from build123d import *

# Parameters (mm, degrees)
F0_W     = 165.1
F0_H     = 304.8
F0_W_2   = 139.7
F0_H_2   = 152.4
F0_W_3   = 127
F0_H_3   = 121.92
F0_W_4   = 88.9
F0_H_4   = 114.3
F1_DEPTH = 50.8
F2_DEPTH = 5
F3_DEPTH = 38.1
F4_R     = 10
F5_R     = 3.81
F6_DEPTH = 129.54


# Not quite as in the source:
# - a feature names something its author has since deleted; it is built from what else it names


with BuildPart() as f1:
    # F0 (on Front) → F1 (new body)
    with BuildSketch(Plane.XZ):
        with Locations((0, -38.1)):
            Rectangle(F0_W, F0_H)
        Rectangle(F0_W_2, F0_H_2, mode=Mode.SUBTRACT)
        Rectangle(F0_W_2, F0_H_2)
        Rectangle(F0_W_3, F0_H_3, mode=Mode.SUBTRACT)
        Rectangle(F0_W_3, F0_H_3)
        Rectangle(F0_W_4, F0_H_4, mode=Mode.SUBTRACT)
    extrude(amount=-F1_DEPTH)

    # F0 (on Front) → F2 (cut)
    with BuildSketch(Plane.XZ):
        Rectangle(F0_W_2, F0_H_2)
        Rectangle(F0_W_3, F0_H_3, mode=Mode.SUBTRACT)
    extrude(amount=-F2_DEPTH, mode=Mode.SUBTRACT)

    # F0 (on Front) → F3 (cut)
    with BuildSketch(Plane.XZ):
        Rectangle(F0_W_3, F0_H_3)
        Rectangle(F0_W_4, F0_H_4, mode=Mode.SUBTRACT)
    extrude(amount=-F3_DEPTH, mode=Mode.SUBTRACT)

    # F4
    f4_edges = [f1.edges().sort_by_distance(p)[0] for p in [
        (-44.45, 44.45, 57.15),
        (44.45, 44.45, 57.15),
        (-44.45, 44.45, -57.15),
        (44.45, 44.45, -57.15),
    ]]
    fillet(f4_edges, radius=F4_R)

    # F5 (on face) → F6 (cut, through all)
    with BuildSketch(Plane.XY.offset(-60.96)):
        with Locations((-53.5, 19.05)):
            Circle(F5_R)
        with Locations((53.4924, 19.05)):
            Circle(F5_R)
    extrude(amount=-F6_DEPTH, mode=Mode.SUBTRACT)


solid = f1.part
Source: CAD feature listing. Evaluate the final solid. Frame: model axes, mm. A direction names the side the tool comes from. Round coordinates to 2 decimals unless told otherwise and drop trailing zeros. Loops run counter-clockwise (first coordinate to the right, second up) from the corner with the lowest first, then second, coordinate; pieces in that order, holes last.
Q1. First-contact query: P1, Ø2, axis at x = -63.5, z = -65, coming from the -Y side. Flat tip, straight axial feed; report the tip coordinate or a pass-through.
Q2. Section A-A, the plane z = -41. Return loops of the section in (x, y).
Q3. Section D-D, the plane z = 65. Return loops of the section in (x, y), plus the area to 3 significant figures.
Q4. Section C-C, the plane y = 32.5. Return loops of the section in (x, z).
Q5. Mould query, pull axis X, two halves, no side actions, for faces 1 (the face through (-1, 25, 114.3)), 2 (the face through (-41.44, 44.54, -54.3)), 3 (the face through (-82.55, 25, -40)), 4 (the face through (82.55, 25, -40)). Classes: pulls with the +X half, pulls with the -X half, needs draft (parallel to the pull), parting line crosses it, or undercut.
Q6. Section B-B, the plane x = 10.5. Return loops of the section in (y, z), plus the area to 3 significant figures.
Q7. Access query for faces 5 (the face through (57.126, 20.194, -124.823)), 6 (the face through (-47, 38.1, 5)), 7 (the face through (-1, 50.8, -70)), 8 (the face through (44.45, 44, -1)). Directions: +Z, -Z, +X, -X, +Y, -Y. A direction counts if a zero-diameter tool reaches every point of the face in a straight line with its end or side. Return the directions, or none.
Q8. Ray query, line 1 (Z direction, x = -42.5, y = 17.5); line 2 (X direction, y = 31, z = -6.5); line 3 (Z direction, x = 10, y = 39). Return the intervals inside material, ascending.
Solutions:
1. P1: stops at y = 5
2. outline: (-82.55, 0) - (-69.85, 0) - (-69.85, 5) - (-63.5, 5) - (-63.5, 38.1) - (-44.45, 38.1) - (-44.45, 50.8) - (-82.55, 50.8) - close; (44.45, 38.1) - (63.5, 38.1) - (63.5, 5) - (69.85, 5) - (69.85, 0) - (82.55, 0) - (82.55, 50.8) - (44.45, 50.8) - close
3. outline: (-82.55, 0) - (-69.85, 0) - (-69.85, 5) - (69.85, 5) - (69.85, 0) - (82.55, 0) - (82.55, 50.8) - (-82.55, 50.8) - close
3. area: 7,690 mm2
4. outline: (-82.55, -190.5) - (82.55, -190.5) - (82.55, 114.3) - (-82.55, 114.3) - close; hole (-63.5, -60.96) - (63.5, -60.96) - (63.5, 60.96) - (-63.5, 60.96) - close
5. face 1: needs draft
5. face 2: undercut
5. face 3: pulls with the -X half
5. face 4: pulls with the +X half
6. outline: (0, -190.5) - (50.8, -190.5) - (50.8, -57.15) - (38.1, -57.15) - (38.1, -60.96) - (5, -60.96) - (5, -76.2) - (0, -76.2) - close; (0, 76.2) - (5, 76.2) - (5, 60.96) - (38.1, 60.96) - (38.1, 57.15) - (50.8, 57.15) - (50.8, 114.3) - (0, 114.3) - close
6. area: 9,230 mm2
7. face 5: -Z
7. face 6: -Y
7. face 7: +Z, -Z, +X, -X, +Y
7. face 8: +Y, -Y
8. line 1: z = -190.5 to -60.96, 60.96 to 114.3
8. line 2: x = -82.55 to -63.5, 63.5 to 82.55
8. line 3: z = -190.5 to -57.15, 57.15 to 114.3
